```python
from build123d import *

# Parameters (mm, degrees)
SKETCH_1_R      = 5.1
SKETCH_1_R_2    = 1.6
SKETCH_1_R_3    = 1.1
EXTRUDE_1_DEPTH = 2


with BuildPart() as part:
    # ｽｹｯﾁ1 → ﾎﾞｽ - 押し出し1 (new body)
    with BuildSketch(Plane(origin=(0, 0, 0), x_dir=(0, 0, -1), z_dir=(1, 0, 0))):
        with BuildLine():
            Line((-4.330127019, 20), (-19.485571585, -6.25))
            ThreePointArc((-19.485571585, -6.25), (-19.485571585, -11.25), (-15.155444566, -13.75))
            Line((-15.155444566, -13.75), (15.155444566, -13.75))
            ThreePointArc((15.155444566, -13.75), (19.485571585, -11.25), (19.485571585, -6.25))
            Line((19.485571585, -6.25), (4.330127019, 20))
            ThreePointArc((4.330127019, 20), (0, 22.5), (-4.330127019, 20))
        make_face()
        Circle(SKETCH_1_R, mode=Mode.SUBTRACT)
        with Locations((0, 17.5)):
            Circle(SKETCH_1_R_2, mode=Mode.SUBTRACT)
        with Locations((-8.5, 0)):
            Circle(SKETCH_1_R_3, mode=Mode.SUBTRACT)
        with Locations(Location((8.5, 0, 0), (0, 0, 180))):
            Circle(SKETCH_1_R_3, mode=Mode.SUBTRACT)
        with Locations((15.155444566, -8.75)):
            Circle(SKETCH_1_R_2, mode=Mode.SUBTRACT)
        with BuildLine():
            ThreePointArc((-15.891264638, -7.329236536), (-16.541085212, -9.55), (-14.292937349, -10.097620607))
            ThreePointArc((-14.292937349, -10.097620607), (-13.76980392, -7.95), (-15.891264638, -7.329236536))
        make_face(mode=Mode.SUBTRACT)
    extrude(amount=EXTRUDE_1_DEPTH)


solid = part.part
```
Could you check a few things on this model? Use its own coordinates, in mm. Coordinates: 2 decimals unless noted, no trailing zeros. Write each loop counter-clockwise with the first axis right and the second up, starting at its lowest first coordinate (ties: lowest second). Pieces come first, ordered by that corner, then holes. Notation, with made-up numbers: (83, -16.75) -> (97, -16.75) arc R29 ccw to (97, 17.25) -> close; hole circle Ø2 at (54.25, -33). An arc over 180 degrees is marked (long way). One line per question, with ' | ' between items. Start each with the question number.
1. Thinking about a two-plate mould opening in Z: for faces 1 (the face through (0.99, -11.31, -19.45)), 2 (the face through (0.986, -0.421, 7.484)), 3 (the face through (0, -3.4, -4.2)), which applies, pulls with the +Z half, pulls with the -Z half, needs draft (parallel to the pull), parting line crosses it, or undercut?
2. If we section it at C-C (y = 2): Please give me the cut outline in (x, z).
3. If we section it at A-A (z = 0): Please give me the cut outline in (x, y), and give its area (3 significant figures).
4. Will this pin go through, and if not, where does the flat tip stop? P1, Ø2.5, axis at y = 17.5, z = 0, coming from the +X side.
5. Please list where these lines run through material, in increasing order: line 1 along Y through (x, z) = (1.1, 4); line 2 along Z through (x, y) = (1.15, 0.5); line 3 along Y through (x, z) = (1.85, 16.5).
6. If we section it at D-D (x = 1): Please give me the cut outline in (y, z).
7. If we section it at B-B (y = -8.75): Please give me the cut outline in (x, z), and give its area (3 significant figures).
Return value:
1) face 1: pulls with the -Z half | face 2: undercut | face 3: needs draft
2) outline: (0, -14.72) -> (2, -14.72) -> (2, -4.69) -> (0, -4.69) -> close; (0, 4.69) -> (2, 4.69) -> (2, 14.72) -> (0, 14.72) -> close
3) outline: (0, -13.75) -> (2, -13.75) -> (2, -5.1) -> (0, -5.1) -> close; (0, 5.1) -> (2, 5.1) -> (2, 15.9) -> (0, 15.9) -> close; (0, 19.1) -> (2, 19.1) -> (2, 22.5) -> (0, 22.5) -> close | area: 45.7 mm²
4) P1: passes through
5) line 1: y = -13.75 to -3.16, 3.16 to 20.5 | line 2: z = -15.59 to -9.48, -7.52 to -5.08, 5.08 to 7.52, 9.48 to 15.59 | line 3: y = -13.57 to -9.62, -7.88 to -1.08
6) outline: (-13.75, -15.16) arc R5 ccw to (-6.25, -19.49) -> (20, -4.33) arc R5 ccw to (20, 4.33) -> (-6.25, 19.49) arc R5 ccw to (-13.75, 15.16) -> close; hole circle Ø3.2 at (-8.75, -15.16); hole circle Ø3.2 at (-8.75, 15.16); hole circle Ø10.2 at (0, 0); hole circle Ø2.2 at (0, -8.5); hole circle Ø2.2 at (0, 8.5); hole circle Ø3.2 at (17.5, 0)
7) outline: (0, -20.16) -> (2, -20.16) -> (2, -16.76) -> (0, -16.76) -> close; (0, -13.56) -> (2, -13.56) -> (2, 13.56) -> (0, 13.56) -> close; (0, 16.76) -> (2, 16.76) -> (2, 20.16) -> (0, 20.16) -> close | area: 67.8 mm²
